Print and shaded views of the part. All mm, measured from the part's lowest x, y and z. A direction names the side the tool comes from. Give positions to 0.01 mm unless a question says otherwise; leave off trailing zeros. Write each loop counter-clockwise with the first axis right and the second up, starting at its lowest first coordinate (ties: lowest second). Pieces come first, ordered by that corner, then holes.
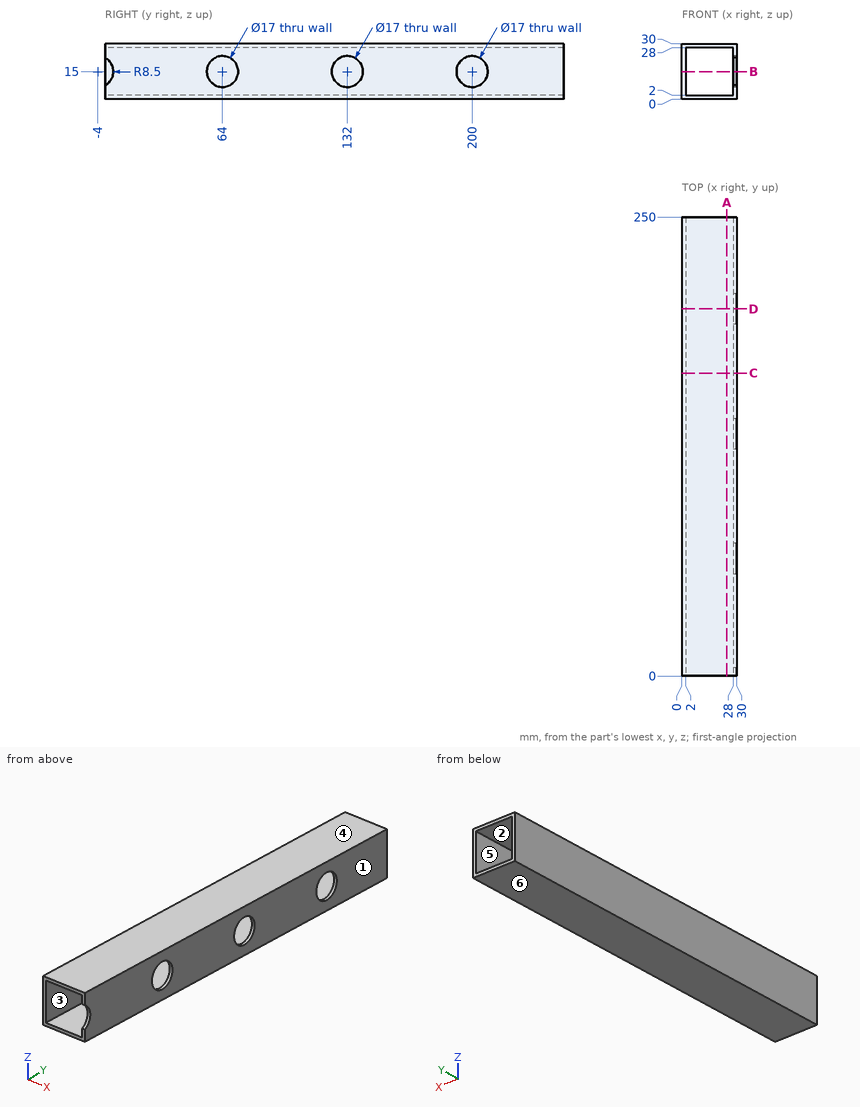
1. Drop flat-ended pins along their axis: pin 1 (12 mm diameter, centred on x = 21, z = 12.5, fed in from +Y); pin 2 (13.5 mm diameter, centred on y = 132, z = 15, fed in from +X). Give the stop position or say it passes through.
2. 3-axis set-ups, long thin cutter, end or side, ignore diameter. For the marked faces 1 and 2: which of +Z, -Z, +X, -X, +Y, -Y reach the whole face in a straight line?
3. Saw through at D-D on y = 200. Give the cut face in (x, z).
4. Saw through at B-B on z = 15. Give the cut face in (x, y).
5. Saw through at C-C on y = 165. Give the cut face in (x, z), plus the area to 3 significant figures.
6. Mould opens along Z. For the marked faces 3, 4, 5 and 6 say: pulls with the +Z half, pulls with the -Z half, needs draft (parallel to the pull), parting line crosses it, or undercut.
7. Saw through at A-A on x = 24.5. Give the cut face in (y, z).
8. Drill centre lines: line 1 along Y through (x, z) = (29.2, 15); line 2 along Z through (x, y) = (11.25, 181.5). Where is each one in solid material? Low to high.
Outcome:
1. pin 1: passes through
1. pin 2: stops at x = 2
2. face 1: +Z, -Z, +X, +Y, -Y
2. face 2: +Y, -Y
3. outline: (0, 0) - (30, 0) - (30, 6.5) - (28, 6.5) - (28, 2) - (2, 2) - (2, 28) - (28, 28) - (28, 23.5) - (30, 23.5) - (30, 30) - (0, 30) - close
4. outline: (0, 0) - (2, 0) - (2, 250) - (0, 250) - close; (28, 4.5) - (30, 4.5) - (30, 55.5) - (28, 55.5) - close; (28, 72.5) - (30, 72.5) - (30, 123.5) - (28, 123.5) - close; (28, 140.5) - (30, 140.5) - (30, 191.5) - (28, 191.5) - close; (28, 208.5) - (30, 208.5) - (30, 250) - (28, 250) - close
5. outline: (0, 0) - (30, 0) - (30, 30) - (0, 30) - close; hole (2, 2) - (28, 2) - (28, 28) - (2, 28) - close
5. area: 224 mm2
6. face 3: undercut
6. face 4: pulls with the +Z half
6. face 5: undercut
6. face 6: pulls with the -Z half
7. outline: (0, 0) - (250, 0) - (250, 2) - (0, 2) - close; (0, 28) - (250, 28) - (250, 30) - (0, 30) - close
8. line 1: y = 4.5 to 55.5, 72.5 to 123.5, 140.5 to 191.5, 208.5 to 250
8. line 2: z = 0 to 2, 28 to 30
